from build123d import *

# Parameters (mm, degrees)
SKETCH1_W           = 19
SKETCH1_H           = 6
SKETCH1_W_2         = 9.5
SKETCH1_H_2         = 9
BOSS_EXTRUDE1_DEPTH = 120
SKETCH2_R           = 1.7
SKETCH2_R_2         = 1.55
CUT_EXTRUDE1_DEPTH  = 19


with BuildPart() as part:
    # Sketch1 → Boss-Extrude1 (new body)
    with BuildSketch(Plane(origin=(0, 0, 0), x_dir=(1, 0, 0), z_dir=(0, 1, 0))):
        Rectangle(SKETCH1_W, SKETCH1_H)
        with Locations((-4.75, 7.5)):
            Rectangle(SKETCH1_W_2, SKETCH1_H_2)
    extrude(amount=BOSS_EXTRUDE1_DEPTH)

    # Sketch2 → Cut-Extrude1 (cut)
    with BuildSketch(Plane(origin=(9.5, 0, -9.5), x_dir=(0, 0, 1), z_dir=(-1, 0, 0))):
        with Locations(Location((9.670877536, 111, 0), (0, 0, 180))):
            Circle(SKETCH2_R)
        with Locations(Location((9.670877536, 82.75, 0), (0, 0, 180))):
            Circle(SKETCH2_R)
        with Locations(Location((9.670877536, 37.25, 0), (0, 0, 180))):
            Circle(SKETCH2_R)
        with Locations(Location((9.670877536, 9, 0), (0, 0, 180))):
            Circle(SKETCH2_R)
        with Locations(Location((9.370877536, 91.5, 0), (0, 0, 180))):
            Circle(SKETCH2_R_2)
        with Locations(Location((9.370877536, 74, 0), (0, 0, 180))):
            Circle(SKETCH2_R_2)
    extrude(amount=CUT_EXTRUDE1_DEPTH, mode=Mode.SUBTRACT)


solid = part.part
The listing builds one solid part. Answer for the finished solid, in the listing's coordinates (mm). A direction names the side the tool comes from. Give positions to 0.01 mm unless a question says otherwise; leave off trailing zeros. Write each loop counter-clockwise with the first axis right and the second up, starting at its lowest first coordinate (ties: lowest second). Pieces come first, ordered by that corner, then holes. Notation, with made-up numbers: (-24, 40.5) -> (9, 40.5) arc R26 cw to (9, 60.5) -> close; hole circle Ø5 at (85, 41.5). An arc over 180 degrees is marked (long way). One line per question, with ' | ' between items. Start each with the question number.
1. Find the intervals of material crossed by probe 1 along Z at (x, y) = (-5, 82.75); probe 2 along Z at (x, y) = (-1.5, 91.5); probe 3 along X at (y, z) = (79, -5.75), in increasing order.
2. Section A-A (x = -4) is taken. Determine the outline of the cut face in (y, z).
3. Section B-B (y = 74) is taken. Determine the outline of the cut face in (x, z).
4. Given pin 1 Ø4.5 at (y, z) = (81.5, -6.5) entering from +X; pin 2 Ø2 at (x, z) = (-2.5, -5) entering from -Y; pin 3 Ø7.5 at (x, y) = (5, 54.5) entering from -Z, each flat-ended and moving along its own axis, determine where each tip first touches the part or whether it passes through.
5. For a pull along Y with two mould halves and no side action, classify faces 1 (the flat face through (5, 59, -3)), 2 (the cylindrical face through (0.133, 89.963, 0.073)), 3 (the flat face through (-2, 120, -3)) as pulls with the +Y half, pulls with the -Y half, needs draft (parallel to the pull), parting line crosses it, or undercut.
6. Section D-D (z = -7.5) is taken. Determine the outline of the cut face in (x, y), plus the area to 3 significant figures.
7. For faces 4 (the cylindrical face through (0.13, 10.66, 0.54)), 5 (the flat face through (0, 59, -7)), determine the directions among +Z, -Z, +X, -X, +Y, -Y from which every point of the face is accessible in a straight line to the end or side of a thin tool.
8. Section C-C (y = 111) is taken. Determine the outline of the cut face in (x, z), plus the area to 3 significant figures.
Response values:
1) probe 1: -12 to -1.53, 1.87 to 3 | probe 2: -12 to -1.68, 1.42 to 3 | probe 3: -9.5 to 0
2) outline: (0, -12) -> (120, -12) -> (120, 3) -> (0, 3) -> close; hole circle Ø3.4 at (9, 0.17); hole circle Ø3.4 at (37.25, 0.17); hole circle Ø3.1 at (74, -0.13); hole circle Ø3.4 at (82.75, 0.17); hole circle Ø3.1 at (91.5, -0.13); hole circle Ø3.4 at (111, 0.17)
3) outline: (-9.5, -12) -> (0, -12) -> (0, -3) -> (9.5, -3) -> (9.5, -1.68) -> (-9.5, -1.68) -> close; (-9.5, 1.42) -> (9.5, 1.42) -> (9.5, 3) -> (-9.5, 3) -> close
4) pin 1: x = 0 | pin 2: y = 0 | pin 3: z = -3
5) face 1: needs draft | face 2: undercut | face 3: pulls with the +Y half
6) outline: (-9.5, 0) -> (0, 0) -> (0, 120) -> (-9.5, 120) -> close | area: 1,140 mm2
7) face 4: +X, -X | face 5: -Z, +X, +Y, -Y
8) outline: (-9.5, -12) -> (0, -12) -> (0, -3) -> (9.5, -3) -> (9.5, -1.53) -> (-9.5, -1.53) -> close; (-9.5, 1.87) -> (9.5, 1.87) -> (9.5, 3) -> (-9.5, 3) -> close | area: 135 mm2
